Verification items for the finished model (mm, model axes). A direction names the side the tool comes from. Give positions to 0.01 mm unless a question says otherwise; leave off trailing zeros. Order: outer loops, then holes, each group sorted by start corner. A loop starts at its lowest first (then second) coordinate and runs counter-clockwise, first axis right, second up.
from build123d import *

# Parameters (mm, degrees)
MASTEREXTRUSION_EXTRUDE1_OUTLINE_W   = 44.45
MASTEREXTRUSION_EXTRUDE1_OUTLINE_H   = 31.75
MASTEREXTRUSION_EXTRUDE1_DEPTH       = 380
EXTRUDE1_DEPTH                       = 382.324091161
MASTEREXTRUSION_START                = 15.875
MASTEREXTRUSION_DEPTH                = 3.175
EXTRUDE3_DEPTH                       = 382.324091161
EXTRUDE3_DEPTH_BACK                  = 382.324091161
BUSHING_HOLES_MASTEREXTRUSION_2_R    = 3
EXTRUDE4_DEPTH                       = 382.324091161
EXTRUDE4_DEPTH_BACK                  = 382.324091161
MOTOR_MOUNTS_MASTEREXTRUSION_2_R     = 11.3109375
MOTOR_MOUNTS_MASTEREXTRUSION_2_R_2   = 0.889
EXTRUDE5_DEPTH                       = 382.324091161
EXTRUDE5_DEPTH_BACK                  = 382.324091161
SKETCH7_MASTEREXTRUSION_2_R          = 2.5527
Z_MOUNTING_HOLES_MASTEREXTRUSION_3_R = 2.5
EXTRUDE7_DEPTH                       = 382.324091161


# Read off the part's stored shape, not the designer's step: <MasterExtrusion>-<Extrude1>, MasterExtrusion
with BuildPart() as part:
    # <MasterExtrusion>-<Extrude1> outline → <MasterExtrusion>-<Extrude1> (new body)
    with BuildSketch(Plane.YZ):
        with BuildLine():
            ThreePointArc((25.4, 15.875), (24.47006403, 18.12006403), (22.225, 19.05))
            Line((22.225, 19.05), (-22.225, 19.05))
            ThreePointArc((-22.225, 19.05), (-24.47006403, 18.12006403), (-25.4, 15.875))
            Line((-25.4, 15.875), (-25.4, -15.875))
            ThreePointArc((-25.4, -15.875), (-24.47006403, -18.12006403), (-22.225, -19.05))
            Line((-22.225, -19.05), (22.225, -19.05))
            ThreePointArc((22.225, -19.05), (24.47006403, -18.12006403), (25.4, -15.875))
            Line((25.4, -15.875), (25.4, 15.875))
        make_face()
        Rectangle(MASTEREXTRUSION_EXTRUDE1_OUTLINE_W, MASTEREXTRUSION_EXTRUDE1_OUTLINE_H, mode=Mode.SUBTRACT)
    extrude(amount=MASTEREXTRUSION_EXTRUDE1_DEPTH)

    # Track-MasterExtrusion<2> → Extrude1 (cut, through all)
    with BuildSketch(Plane.XY):
        with BuildLine():
            Line((54, -3.96), (326, -3.96))
            ThreePointArc((326, -3.96), (334, -11.96), (326, -19.96))
            Line((326, -19.96), (54, -19.96))
            ThreePointArc((54, -19.96), (46, -11.96), (54, -3.96))
        make_face()
    extrude(amount=-EXTRUDE1_DEPTH, mode=Mode.SUBTRACT)

    # MasterExtrusion outline → MasterExtrusion (cut)
    with BuildSketch(Plane.XY.offset(MASTEREXTRUSION_START)):
        with BuildLine():
            ThreePointArc((261, 19.4), (255.343145751, 17.056854249), (253, 11.4))
            Line((253, 11.4), (253, -11.4))
            ThreePointArc((253, -11.4), (255.343145751, -17.056854249), (261, -19.4))
            Line((261, -19.4), (350, -19.4))
            ThreePointArc((350, -19.4), (355.656854249, -17.056854249), (358, -11.4))
            Line((358, -11.4), (358, 11.4))
            ThreePointArc((358, 11.4), (355.656854249, 17.056854249), (350, 19.4))
            Line((350, 19.4), (261, 19.4))
        make_face()
    extrude(amount=MASTEREXTRUSION_DEPTH, mode=Mode.SUBTRACT)

    # Bushing Holes-MasterExtrusion<2> → Extrude3 (cut, two sides: drawn at the far end of the back side and taken through both)
    with BuildSketch(Plane.XY.offset(-EXTRUDE3_DEPTH_BACK)):
        with Locations((25, -6.16)):
            Circle(BUSHING_HOLES_MASTEREXTRUSION_2_R)
        with Locations((370, -6.16)):
            Circle(BUSHING_HOLES_MASTEREXTRUSION_2_R)
    extrude(amount=EXTRUDE3_DEPTH + EXTRUDE3_DEPTH_BACK, mode=Mode.SUBTRACT)

    # Motor Mounts-MasterExtrusion<2> → Extrude4 (cut, two sides: drawn at the far end of the back side and taken through both)
    with BuildSketch(Plane.XY.offset(-EXTRUDE4_DEPTH_BACK)):
        with Locations((25, -6.16)):
            Circle(MOTOR_MOUNTS_MASTEREXTRUSION_2_R)
        with Locations((3.08, -6.16)):
            Circle(MOTOR_MOUNTS_MASTEREXTRUSION_2_R_2)
        with Locations((25, 15.76)):
            Circle(MOTOR_MOUNTS_MASTEREXTRUSION_2_R_2)
        with Locations((46.92, -6.16)):
            Circle(MOTOR_MOUNTS_MASTEREXTRUSION_2_R_2)
        with Locations((25, -28.08)):
            Circle(MOTOR_MOUNTS_MASTEREXTRUSION_2_R_2)
    extrude(amount=EXTRUDE4_DEPTH + EXTRUDE4_DEPTH_BACK, mode=Mode.SUBTRACT)

    # Sketch7-MasterExtrusion<2> → Extrude5 (cut, two sides: drawn at the far end of the back side and taken through both)
    with BuildSketch(Plane(origin=(0, 0, 0), x_dir=(1, 0, 0), z_dir=(0, 1, 0)).offset(-EXTRUDE5_DEPTH_BACK)):
        with Locations(Location((8.75, 10.05, 0), (0, 0, 90))):
            Circle(SKETCH7_MASTEREXTRUSION_2_R)
        with Locations(Location((28.85, 10.05, 0), (0, 0, 90))):
            Circle(SKETCH7_MASTEREXTRUSION_2_R)
        with Locations(Location((28.85, -10.05, 0), (0, 0, 90))):
            Circle(SKETCH7_MASTEREXTRUSION_2_R)
        with Locations(Location((8.75, -10.05, 0), (0, 0, 90))):
            Circle(SKETCH7_MASTEREXTRUSION_2_R)
        with Locations(Location((351.15, 10.05, 0), (0, 0, 90))):
            Circle(SKETCH7_MASTEREXTRUSION_2_R)
        with Locations(Location((371.25, 10.05, 0), (0, 0, 90))):
            Circle(SKETCH7_MASTEREXTRUSION_2_R)
        with Locations(Location((371.25, -10.05, 0), (0, 0, 90))):
            Circle(SKETCH7_MASTEREXTRUSION_2_R)
        with Locations(Location((351.15, -10.05, 0), (0, 0, 90))):
            Circle(SKETCH7_MASTEREXTRUSION_2_R)
    extrude(amount=EXTRUDE5_DEPTH + EXTRUDE5_DEPTH_BACK, mode=Mode.SUBTRACT)

    # z mounting holes-MasterExtrusion<3> → Extrude7 (cut, through all)
    with BuildSketch(Plane.XY):
        with Locations(Location((60, 15.4, 0), (0, 0, 180))):
            Circle(Z_MOUNTING_HOLES_MASTEREXTRUSION_3_R)
        with Locations(Location((240, 15.4, 0), (0, 0, 180))):
            Circle(Z_MOUNTING_HOLES_MASTEREXTRUSION_3_R)
        with Locations(Location((240, -2.6, 0), (0, 0, 180))):
            Circle(Z_MOUNTING_HOLES_MASTEREXTRUSION_3_R)
        with Locations(Location((60, -2.6, 0), (0, 0, 180))):
            Circle(Z_MOUNTING_HOLES_MASTEREXTRUSION_3_R)
        with Locations(Location((96, 15.4, 0), (0, 0, 180))):
            Circle(Z_MOUNTING_HOLES_MASTEREXTRUSION_3_R)
        with Locations(Location((96, -2.6, 0), (0, 0, 180))):
            Circle(Z_MOUNTING_HOLES_MASTEREXTRUSION_3_R)
    extrude(amount=EXTRUDE7_DEPTH, mode=Mode.SUBTRACT)


solid = part.part
(1) Section check A-A, the plane z = 1. Enter the section's corners in (x, y) (3 decimals).
Solved:
outline: (0, -25.4) - (380, -25.4) - (380, -22.225) - (0, -22.225) - close; (0, 22.225) - (380, 22.225) - (380, 25.4) - (0, 25.4) - close
(2) Section check C-C, the plane x = 340. Enter the section's corners in (y, z) (3 decimals), then the cut area to 3 significant figures.
Solved:
outline: (-25.4, -15.875) arc R3.175 ccw to (-22.225, -19.05) - (22.225, -19.05) arc R3.175 ccw to (25.4, -15.875) - (25.4, 15.875) arc R3.175 ccw to (22.225, 19.05) - (19.4, 19.05) - (19.4, 15.875) - (22.225, 15.875) - (22.225, -15.875) - (-22.225, -15.875) - (-22.225, 15.875) - (-19.4, 15.875) - (-19.4, 19.05) - (-22.225, 19.05) arc R3.175 ccw to (-25.4, 15.875) - close
area: 392 mm2
(3) Go/stop test with flat-tipped pins: pin 1 (10 mm diameter, centred on y = -1, z = -9.5, fed in from -X); pin 2 (1 mm diameter, centred on x = 246, z = -17.5, fed in from -Y); pin 3 (1 mm diameter, centred on x = 316, z = 17.5, fed in from +Y); pin 4 (1.6 mm diameter, centred on x = 150.5, z = -18, fed in from +Y). Record where each tip stops, or that it passes through.
Solved:
pin 1: passes through
pin 2: stops at y = -25.19
pin 3: stops at y = 25.19
pin 4: stops at y = 25.11
(4) Set-up check for faces 4 (the cylindrical face through (255.281, -16.994, 17.44)), 5 (the flat face through (145, 0, 15.875)), 6 (the flat face through (0, 0, 17)), 7 (the flat face through (145, 0, 19.05)), 8 (the cylindrical face through (355.719, 16.994, 17.44)): record each of +Z, -Z, +X, -X, +Y, -Y from which the full face is reachable in a straight line by a thin tool's end or side.
Solved:
face 4: +Z, -Z
face 5: +X, -X
face 6: +Z, -Z, -X, +Y, -Y
face 7: +Z, +X, -X, +Y, -Y
face 8: +Z
(5) Section check D-D, the plane x = 224. Enter the section's corners in (y, z) (3 decimals), then the cut area to 3 significant figures.
Solved:
outline: (-25.4, -15.875) arc R3.175 ccw to (-22.225, -19.05) - (-19.96, -19.05) - (-19.96, -15.875) - (-22.225, -15.875) - (-22.225, 15.875) - (22.225, 15.875) - (22.225, -15.875) - (-3.96, -15.875) - (-3.96, -19.05) - (22.225, -19.05) arc R3.175 ccw to (25.4, -15.875) - (25.4, 15.875) arc R3.175 ccw to (22.225, 19.05) - (-22.225, 19.05) arc R3.175 ccw to (-25.4, 15.875) - close
area: 465 mm2
(6) Release check for a two-part mould opening along Y. For faces 1 (the flat face through (187, 5, -19.05)), 2 (the flat face through (187, -25.4, 0)), 3 (the cylindrical face through (46, -12, -17)) record: pulls with the +Y half, pulls with the -Y half, needs draft (parallel to the pull), parting line crosses it, or undercut.
Solved:
face 1: needs draft
face 2: pulls with the -Y half
face 3: undercut
(7) Section check B-B, the plane x = 281.5. Enter the section's corners in (y, z) (3 decimals).
Solved:
outline: (-25.4, -15.875) arc R3.175 ccw to (-22.225, -19.05) - (-19.96, -19.05) - (-19.96, -15.875) - (-22.225, -15.875) - (-22.225, 15.875) - (-19.4, 15.875) - (-19.4, 19.05) - (-22.225, 19.05) arc R3.175 ccw to (-25.4, 15.875) - close; (-3.96, -19.05) - (22.225, -19.05) arc R3.175 ccw to (25.4, -15.875) - (25.4, 15.875) arc R3.175 ccw to (22.225, 19.05) - (19.4, 19.05) - (19.4, 15.875) - (22.225, 15.875) - (22.225, -15.875) - (-3.96, -15.875) - close
(8) Scan lines: line 1 (X direction, y = -24.5, z = -10.05); line 2 (Y direction, x = 114, z = -3.5) (3 decimals); line 3 (X direction, y = -6.16, z = 17). Record each from-to range of solid material in increasing order.
Solved:
line 1: x = 0 to 6.2, 11.3 to 26.3, 31.4 to 348.6, 353.7 to 368.7, 373.8 to 380
line 2: y = -25.4 to -22.225, 22.225 to 25.4
line 3: x = 0 to 2.19, 3.97 to 13.69, 36.31 to 46.03, 47.81 to 253, 358 to 367, 373 to 380
